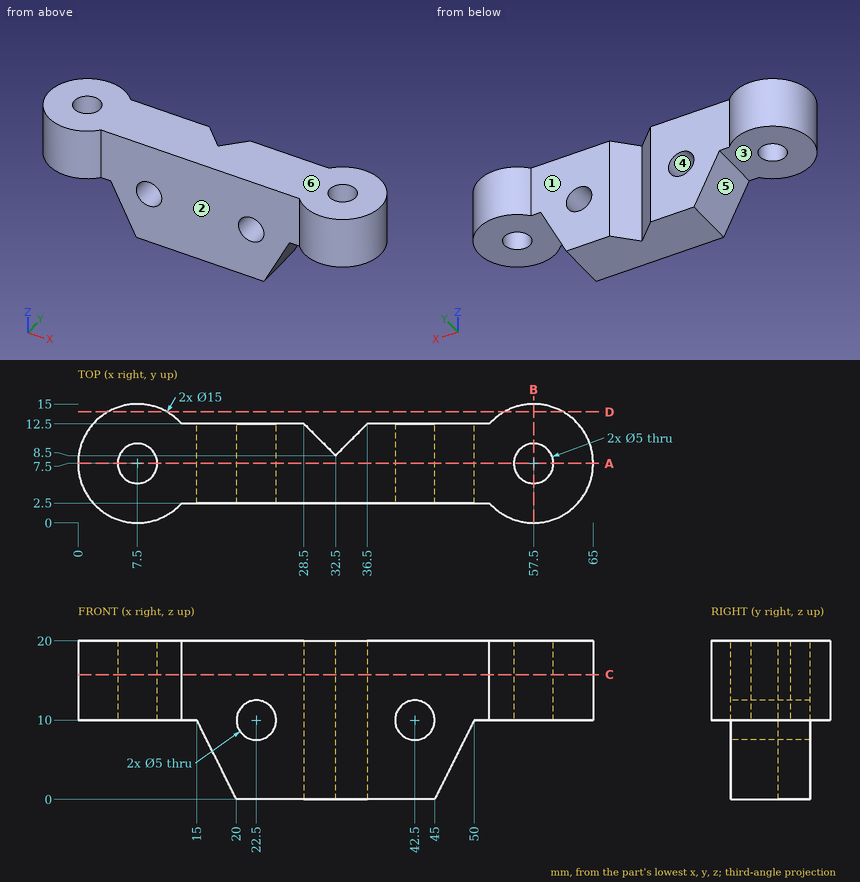
Print and shaded views of the part. All mm, measured from the part's lowest x, y and z. A direction names the side the tool comes from. Round coordinates to 2 decimals unless told otherwise and drop trailing zeros. Write each loop counter-clockwise with the first axis right and the second up, starting at its lowest first coordinate (ties: lowest second). Pieces come first, ordered by that corner, then holes.
(1) Mould opens along X. For the marked faces 4, 5 and 6 say: pulls with the +X half, pulls with the -X half, needs draft (parallel to the pull), parting line crosses it, or undercut.
(2) Probe line 1 along X through (y, z) = (9, 16.5); line 2 along X through (y, z) = (8.25, 16.5) (1 decimal); line 3 along Y through (x, z) = (16, 13.5). List the from-to ranges inside material, lowest first.
(3) 3-axis set-ups, long thin cutter, end or side, ignore diameter. For the marked faces 1, 2 and 3: which of +Z, -Z, +X, -X, +Y, -Y reach the whole face in a straight line?
(4) Slice it at D-D, the plane y = 14. Write the cut outline in (x, z), and give its area (3 significant figures).
(5) Slice it at B-B, the plane x = 57.5. Write the cut outline in (y, z).
(6) Drop flat-ended pins along their axis: P1, Ø6, axis at x = 31.5, z = 11, coming from the -Y side; P2, Ø4, axis at x = 42.5, z = 10, coming from the +Y side; P3, Ø3, axis at y = 11.5, z = 17.5, coming from the +X side; P4, Ø1, axis at x = 15.5, y = 7, coming from the -Z side. Give the stop position or say it passes through.
(7) Slice it at C-C, the plane z = 15.75. Write the cut outline in (x, y).
(8) Slice it at A-A, the plane y = 7.5. Write the cut outline in (x, z), and give its area (3 significant figures).
From the geometry:
1. face 4: undercut
1. face 5: pulls with the -X half
1. face 6: needs draft
2. line 1: x = 0.15 to 5.5, 9.5 to 32, 33 to 55.5, 59.5 to 64.85
2. line 2: x = 0 to 5.1, 9.9 to 55.1, 59.9 to 65
2. line 3: y = 2.5 to 12.5
3. face 1: +Z, -Z, +Y
3. face 2: +Z, -Z, -Y
3. face 3: -Z, -X, +Y, -Y
4. outline: (3.76, 10) - (11.24, 10) - (11.24, 20) - (3.76, 20) - close; (53.76, 10) - (61.24, 10) - (61.24, 20) - (53.76, 20) - close
4. area: 150 mm2
5. outline: (0, 10) - (5, 10) - (5, 20) - (0, 20) - close; (10, 10) - (15, 10) - (15, 20) - (10, 20) - close
6. P1: stops at y = 2.5
6. P2: passes through
6. P3: stops at x = 64.57
6. P4: stops at z = 8
7. outline: (13.09, 2.5) - (51.91, 2.5) arc R7.5 ccw (long way) to (51.91, 12.5) - (36.5, 12.5) - (32.5, 8.5) - (28.5, 12.5) - (13.09, 12.5) arc R7.5 ccw (long way) to start; hole circle Ø5 at (7.5, 7.5); hole circle Ø5 at (57.5, 7.5)
8. outline: (0, 10) - (5, 10) - (5, 20) - (0, 20) - close; (10, 10) - (15, 10) - (20, 0) - (45, 0) - (50, 10) - (55, 10) - (55, 20) - (10, 20) - close; (60, 10) - (65, 10) - (65, 20) - (60, 20) - close; hole circle Ø5 at (22.5, 10); hole circle Ø5 at (42.5, 10)
8. area: 811 mm2
